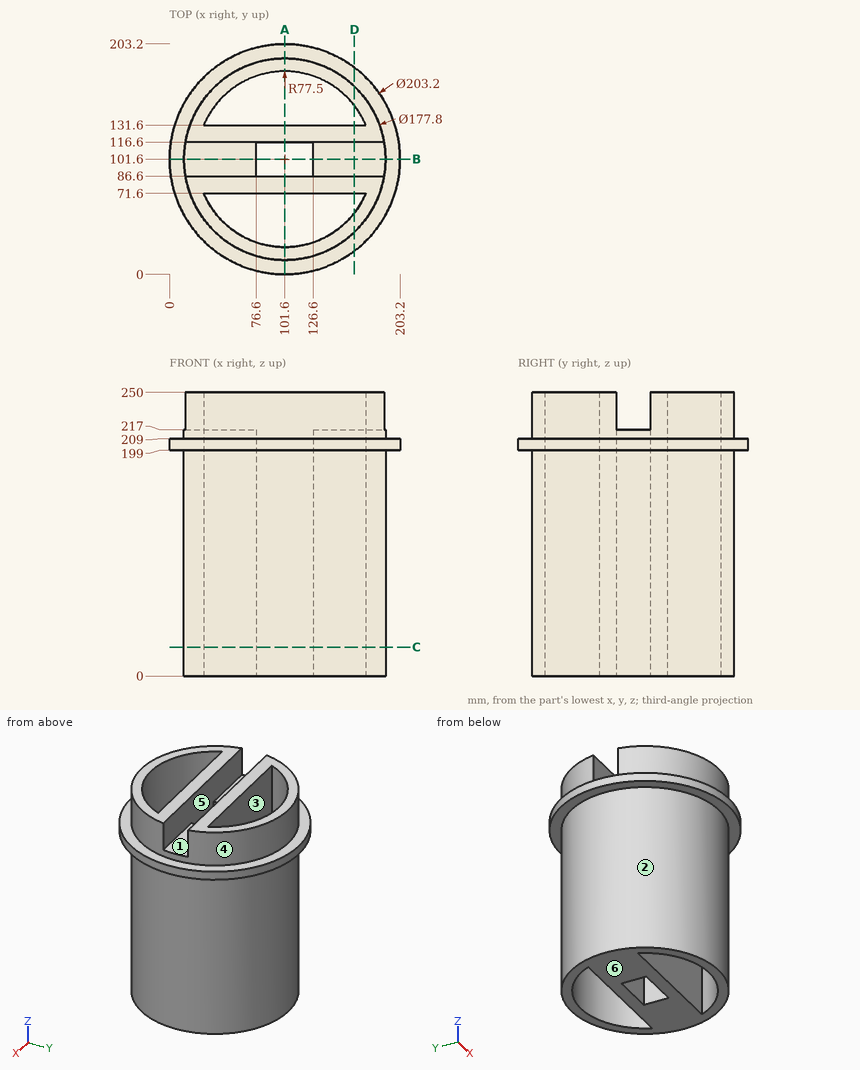
The drawing under review shows one solid part. Ordinate dimensions are in mm from its lowest x, y, z. A direction names the side the tool comes from. Give positions to 0.01 mm unless a question says otherwise; leave off trailing zeros. Write each loop counter-clockwise with the first axis right and the second up, starting at its lowest first coordinate (ties: lowest second). Pieces come first, ordered by that corner, then holes.
1. Draft analysis for pull direction Y (two halves, no side actions). For the marked faces 4, 5 and 6, state which applies: +Y half, -Y half, draft (parallel to the pull), parting line (faces both ways), or undercut.
2. Wall thickness on L1, parallel to Y at x = 154, z = 208.5; L2, parallel to Y at x = 55, z = 134; L3, parallel to Y at x = 88, z = 60: over which ranges is each line inside the solid? List them lowest first.
3. Add section D-D, the plane x = 163. Write out the cut boundary in (y, z).
4. Add section B-B, the plane y = 101.6. Write out the cut boundary in (x, z), plus the area to 3 significant figures.
5. Add section C-C, the plane z = 25.5. Write out the cut boundary in (x, y), plus the area to 3 significant figures.
6. Tool access review of the marked faces 1, 2 and 3: name each direction out of +Z, -Z, +X, -X, +Y, -Y from which nothing blocks a thin tool from reaching the whole face with its end or side.
7. Add section A-A, the plane x = 101.6. Write out the cut boundary in (y, z), plus the area to 3 significant figures.
8. For P1, Ø15, axis at y = 98, z = 137.5, coming from the -X side; P2, Ø10, axis at y = 52.5, z = 55.5, coming from the -X side; P3, Ø6, axis at y = 70.5, z = 104, coming from the -X side, all flat-tipped, find the tip position at first contact; note any pin that passes through.
Worked answers:
1. face 4: parting line
1. face 5: undercut
1. face 6: draft
2. L1: y = 14.56 to 44.5, 71.6 to 131.6, 158.7 to 188.64
2. L2: y = 25.89 to 39.68, 71.6 to 131.6, 163.52 to 177.31
2. L3: y = 13.75 to 25.3, 71.6 to 86.6, 116.6 to 131.6, 177.9 to 189.45
3. outline: (20.65, 199) - (37.31, 199) - (37.31, 0) - (54.31, 0) - (54.31, 250) - (37.31, 250) - (37.31, 209) - (20.65, 209) - close; (71.6, 0) - (131.6, 0) - (131.6, 250) - (116.6, 250) - (116.6, 217) - (86.6, 217) - (86.6, 250) - (71.6, 250) - close; (148.89, 0) - (165.89, 0) - (165.89, 199) - (182.55, 199) - (182.55, 209) - (165.89, 209) - (165.89, 250) - (148.89, 250) - close
4. outline: (0, 199) - (12.7, 199) - (12.7, 0) - (76.6, 0) - (76.6, 217) - (12.7, 217) - (12.7, 209) - (0, 209) - close; (126.6, 0) - (190.5, 0) - (190.5, 199) - (203.2, 199) - (203.2, 209) - (190.5, 209) - (190.5, 217) - (126.6, 217) - close
4. area: 28,000 mm2
5. outline: circle Ø177.8 at (101.6, 101.6); hole (30.14, 71.6) arc R77.5 ccw to (173.06, 71.6) - close; hole (30.14, 131.6) - (173.06, 131.6) arc R77.5 ccw to start; hole (76.6, 86.6) - (126.6, 86.6) - (126.6, 116.6) - (76.6, 116.6) - close
5. area: 13,500 mm2
6. face 1: +Z, +X, -X
6. face 2: -Z
6. face 3: +Z, -Z
7. outline: (0, 199) - (12.7, 199) - (12.7, 0) - (24.1, 0) - (24.1, 250) - (12.7, 250) - (12.7, 209) - (0, 209) - close; (71.6, 0) - (86.6, 0) - (86.6, 250) - (71.6, 250) - close; (116.6, 0) - (131.6, 0) - (131.6, 250) - (116.6, 250) - close; (179.1, 0) - (190.5, 0) - (190.5, 199) - (203.2, 199) - (203.2, 209) - (190.5, 209) - (190.5, 250) - (179.1, 250) - close
7. area: 13,500 mm2
8. P1: stops at x = 12.7
8. P2: stops at x = 24.41
8. P3: stops at x = 17.26
